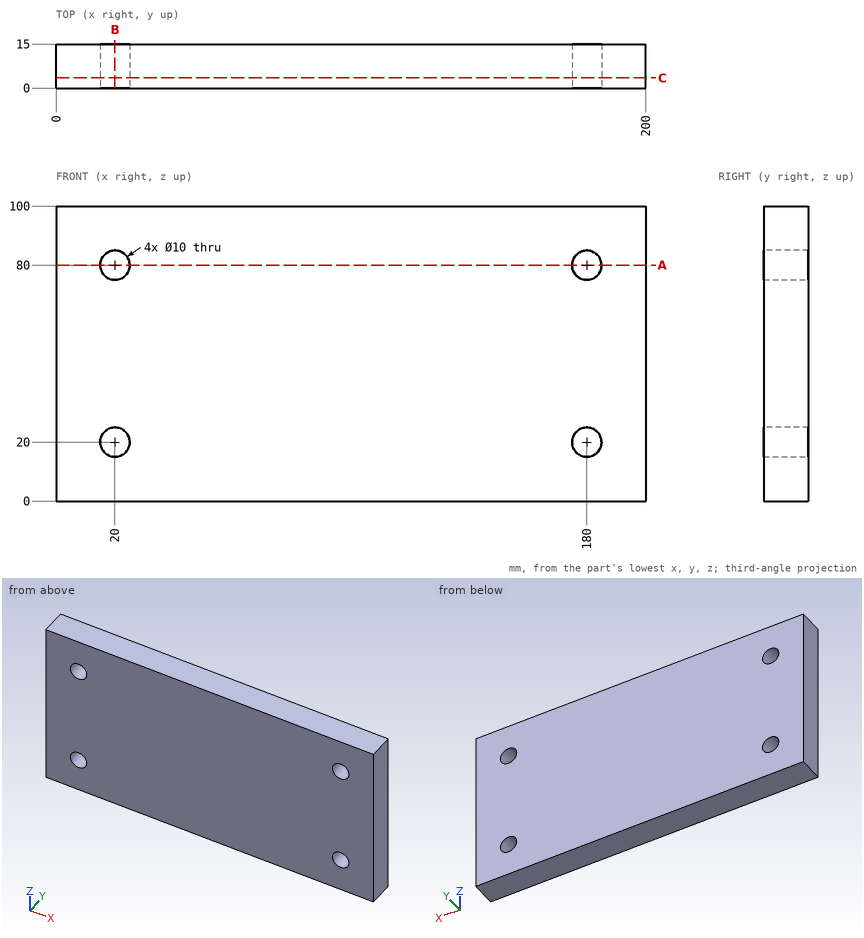
The figure shows three views and two pictorial views of one solid part (mm, origin at its lowest corner). Answer the questions. Round coordinates to 2 decimals unless told otherwise and drop trailing zeros. Order: outer loops, then holes, each group sorted by start corner. A loop starts at its lowest first (then second) coordinate and runs counter-clockwise, first axis right, second up. Notation, with made-up numbers: (-34, 76) -> (-23, 76) arc R27 ccw to (-23, 94) -> close; hole circle Ø9 at (-25, -23.75). An arc over 180 degrees is marked (long way). One line per item, written item: value.
Item 1: Find section B-B, the plane x = 20. Give the vertices of the cut face in (y, z), then the cut area to 3 significant figures.
Taken from the geometry:
outline: (0, 0) -> (15, 0) -> (15, 15) -> (0, 15) -> close; (0, 25) -> (15, 25) -> (15, 75) -> (0, 75) -> close; (0, 85) -> (15, 85) -> (15, 100) -> (0, 100) -> close
area: 1,200 mm2
Item 2: Find section C-C, the plane y = 3.5. Give the vertices of the cut face in (x, z), then the cut area to 3 significant figures.
Taken from the geometry:
outline: (0, 0) -> (200, 0) -> (200, 100) -> (0, 100) -> close; hole circle Ø10 at (20, 20); hole circle Ø10 at (20, 80); hole circle Ø10 at (180, 20); hole circle Ø10 at (180, 80)
area: 19,700 mm2
Item 3: Find section A-A, the plane z = 80. Give the vertices of the cut face in (x, y).
Taken from the geometry:
outline: (0, 0) -> (15, 0) -> (15, 15) -> (0, 15) -> close; (25, 0) -> (175, 0) -> (175, 15) -> (25, 15) -> close; (185, 0) -> (200, 0) -> (200, 15) -> (185, 15) -> close
Item 4: Straight lines are drawn through the part: L1, parallel to Z at x = 180, y = 9.75; L2, parallel to X at y = 11.5, z = 80; L3, parallel to X at y = 8.25, z = 18. For each, find the intervals that lie inside material, in ascending order.
Taken from the geometry:
L1: z = 0 to 15, 25 to 75, 85 to 100
L2: x = 0 to 15, 25 to 175, 185 to 200
L3: x = 0 to 15.42, 24.58 to 175.42, 184.58 to 200
